For this review, take the finished solid that the model builds, in its own axes (mm). A direction names the side the tool comes from. Round coordinates to 2 decimals unless told otherwise and drop trailing zeros. Loops run counter-clockwise (first coordinate to the right, second up) from the corner with the lowest first, then second, coordinate; pieces in that order, holes last.
1) Insertion check: pin 1 (0.5 mm diameter, centred on x = 13.5, y = 1, fed in from -Z); pin 2 (0.5 mm diameter, centred on x = 6, y = 1, fed in from +Z). Each pin has a flat end and moves straight along its axis. Give the tip position at first contact, or say it passes through.
2) Wall thickness on L1, parallel to Z at x = 10, y = 0.8; L2, parallel to Z at x = 12.5, y = 0.5; L3, parallel to Z at x = 9.25, y = 1.35: over which ranges is each line inside the solid? List them lowest first.
3) Mouldability with a two-part tool opening along Z and no side actions: class faces 1 (the flat face through (5, 1, -20)), 2 (the cylindrical face through (17.6, 0.76, -9.95)), 3 (the flat face through (0, 1, -4)) as pulls with the +Z half, pulls with the -Z half, needs draft (parallel to the pull), parting line crosses it, or undercut.
4) Take a section at D-D (z = -10). State the section outline as (x, y) points.
5) Take a section at A-A (y = 1.2). State the section outline as (x, z) points.
6) Tool access review of faces 4 (the flat face through (15, 1, 0)), 5 (the flat face through (15, 1, -20)), 6 (the flat face through (5, 1, 0)): name each direction out of +Z, -Z, +X, -X, +Y, -Y from which nothing blocks a thin tool from reaching the whole face with its end or side.
7) Take a section at B-B (x = 10). State the section outline as (y, z) points.
8) Take a section at C-C (x = 14). State the section outline as (y, z) points.
```python
from build123d import *

# Parameters (mm, degrees)
ESQUISSE1_R        = 1.05
BOSS_EXTRU_1_DEPTH = 1.55


with BuildPart() as part:
    # Esquisse1 → Boss.-Extru.1 (new body)
    with BuildSketch(Plane(origin=(0, 0, 0), x_dir=(1, 0, 0), z_dir=(0, 1, 0))):
        with BuildLine():
            Line((1, 0), (8.2, 0))
            ThreePointArc((8.2, 0), (10, -1.8), (11.8, 0))
            Line((11.8, 0), (19, 0))
            ThreePointArc((19, 0), (19.707106781, 0.292893219), (20, 1))
            Line((20, 1), (20, 7.6))
            ThreePointArc((20, 7.6), (17.6, 10), (20, 12.4))
            Line((20, 12.4), (20, 19))
            ThreePointArc((20, 19), (19.707106781, 19.707106781), (19, 20))
            Line((19, 20), (11.8, 20))
            ThreePointArc((11.8, 20), (10, 21.8), (8.2, 20))
            Line((8.2, 20), (1, 20))
            ThreePointArc((1, 20), (0.292893219, 19.707106781), (0, 19))
            Line((0, 19), (0, 12.4))
            ThreePointArc((0, 12.4), (2.4, 10), (0, 7.6))
            Line((0, 7.6), (0, 1))
            ThreePointArc((0, 1), (0.292893219, 0.292893219), (1, 0))
        make_face()
        with Locations(Location((10, 0, 0), (0, 0, 90))):
            Circle(ESQUISSE1_R, mode=Mode.SUBTRACT)
        with Locations(Location((10, 20, 0), (0, 0, 90))):
            Circle(ESQUISSE1_R, mode=Mode.SUBTRACT)
    extrude(amount=BOSS_EXTRU_1_DEPTH)


solid = part.part
```
Response:
1. pin 1: stops at z = -20
1. pin 2: stops at z = 0
2. L1: z = -21.8 to -21.05, -18.95 to -1.05, 1.05 to 1.8
2. L2: z = -20 to 0
2. L3: z = -21.64 to -20.73, -19.27 to -0.73, 0.73 to 1.64
3. face 1: pulls with the -Z half
3. face 2: undercut
3. face 3: needs draft
4. outline: (2.4, 0) - (17.6, 0) - (17.6, 1.55) - (2.4, 1.55) - close
5. outline: (0, -19) arc R1 ccw to (1, -20) - (8.2, -20) arc R1.8 ccw to (11.8, -20) - (19, -20) arc R1 ccw to (20, -19) - (20, -12.4) arc R2.4 cw to (20, -7.6) - (20, -1) arc R1 ccw to (19, 0) - (11.8, 0) arc R1.8 ccw to (8.2, 0) - (1, 0) arc R1 ccw to (0, -1) - (0, -7.6) arc R2.4 cw to (0, -12.4) - close; hole circle Ø2.1 at (10, -20); hole circle Ø2.1 at (10, 0)
6. face 4: +Z, +X, +Y, -Y
6. face 5: -Z, +X, +Y, -Y
6. face 6: +Z, -X, +Y, -Y
7. outline: (0, -21.8) - (1.55, -21.8) - (1.55, -21.05) - (0, -21.05) - close; (0, -18.95) - (1.55, -18.95) - (1.55, -1.05) - (0, -1.05) - close; (0, 1.05) - (1.55, 1.05) - (1.55, 1.8) - (0, 1.8) - close
8. outline: (0, -20) - (1.55, -20) - (1.55, 0) - (0, 0) - close
